```python
from build123d import *

# Parameters (mm, degrees)
BOSS_EXTRUDE2_DEPTH     = 12
CUT_EXTRUDE1_DEPTH      = 13
SKETCH3_R               = 1.25
CUT_EXTRUDE2_DEPTH      = 13
SKETCH5_R               = 1.65
CUT_EXTRUDE3_DEPTH      = 6
SKETCH6_W               = 12
SKETCH6_H               = 6
CUT_EXTRUDE4_DEPTH      = 13
SKETCH8_W               = 64
SKETCH8_H               = 8
BOSS_EXTRUDE3_DEPTH     = 5
SKETCH9_R               = 1.65
CUT_EXTRUDE5_DEPTH      = 5
SKETCH10_R              = 2
CUT_EXTRUDE6_DEPTH      = 2.5
CUT_EXTRUDE7_DEPTH      = 71.896039473
CUT_EXTRUDE7_DEPTH_BACK = 10


with BuildPart() as part:
    # Sketch1 → Boss-Extrude2 (new body)
    with BuildSketch(Plane.XY):
        with BuildLine():
            Line((0, 0), (64, 0))
            Line((64, 0), (71.941945847, 6.076635266))
            Line((71.941945847, 6.076635266), (89.619615377, 23.754304796))
            ThreePointArc((89.619615377, 23.754304796), (95.283552654, 63.552389681), (55.861435714, 71.4177849))
            Line((55.861435714, 71.4177849), (-7.778174593, 7.778174593))
            Line((-7.778174593, 7.778174593), (0, 0))
        make_face()
    extrude(amount=BOSS_EXTRUDE2_DEPTH)

    # Sketch2 → Cut-Extrude1 (cut, through all)
    with BuildSketch(Plane.XY.offset(12)):
        Polygon((56.718479601, 14.889386235), (39.391727984, 32.210866495), (71.348091567, 64.176955192), (88.674843183, 46.855474932), align=None)
    extrude(amount=-CUT_EXTRUDE1_DEPTH, mode=Mode.SUBTRACT)

    # Sketch3 → Cut-Extrude2 (cut, through all)
    with BuildSketch(Plane.XY.offset(12)):
        with Locations((85.317188693, 39.60711951)):
            Circle(SKETCH3_R)
        with Locations((73.296373413, 27.58630423)):
            Circle(SKETCH3_R)
        with Locations((61.275558133, 15.565488949)):
            Circle(SKETCH3_R)
        with Locations((64.100758142, 60.817095339)):
            Circle(SKETCH3_R)
        with Locations((52.083601094, 48.792622939)):
            Circle(SKETCH3_R)
        with Locations((40.066444047, 36.76815054)):
            Circle(SKETCH3_R)
    extrude(amount=-CUT_EXTRUDE2_DEPTH, mode=Mode.SUBTRACT)

    # Sketch5 → Cut-Extrude3 (cut)
    with BuildSketch(Plane.XZ):
        with Locations((11.5, 6)):
            Circle(SKETCH5_R)
        with Locations((52.5, 6)):
            Circle(SKETCH5_R)
    extrude(amount=-CUT_EXTRUDE3_DEPTH, mode=Mode.SUBTRACT)

    # Sketch6 → Cut-Extrude4 (cut, through all)
    with BuildSketch(Plane.XY.offset(12)):
        with Locations((12, 9)):
            Rectangle(SKETCH6_W, SKETCH6_H)
        with Locations((52, 9)):
            Rectangle(SKETCH6_W, SKETCH6_H)
    extrude(amount=-CUT_EXTRUDE4_DEPTH, mode=Mode.SUBTRACT)

    # Sketch8 → Boss-Extrude3 (add)
    with BuildSketch(Plane.XZ):
        with Locations((32, 16)):
            Rectangle(SKETCH8_W, SKETCH8_H)
    extrude(amount=-BOSS_EXTRUDE3_DEPTH)

    # Sketch9 → Cut-Extrude5 (cut)
    with BuildSketch(Plane.XZ):
        with Locations((11.5, 16)):
            Circle(SKETCH9_R)
        with Locations((52.5, 16)):
            Circle(SKETCH9_R)
    extrude(amount=-CUT_EXTRUDE5_DEPTH, mode=Mode.SUBTRACT)

    # Sketch10 → Cut-Extrude6 (cut)
    with BuildSketch(Plane.XY.offset(12)):
        with Locations((85.317188693, 39.60711951)):
            Circle(SKETCH10_R)
        with Locations((73.296373413, 27.58630423)):
            Circle(SKETCH10_R)
        with Locations((61.275558133, 15.565488949)):
            Circle(SKETCH10_R)
        with Locations((40.060741262, 36.78030582)):
            Circle(SKETCH10_R)
        with Locations((52.081556543, 48.8011211)):
            Circle(SKETCH10_R)
        with Locations((64.102371823, 60.82193638)):
            Circle(SKETCH10_R)
    extrude(amount=-CUT_EXTRUDE6_DEPTH, mode=Mode.SUBTRACT)

    # Sketch11 → Cut-Extrude7 (cut, two sides)
    with BuildSketch(Plane(origin=(0, 5, 0), x_dir=(1, 0, 0), z_dir=(0, 1, 0))) as cut_extrude7_sk:
        with BuildLine():
            ThreePointArc((45, -20), (32, -14.615223689), (19, -20))
            Line((19, -20), (45, -20))
        make_face()
    extrude(amount=CUT_EXTRUDE7_DEPTH, mode=Mode.SUBTRACT)
    extrude(cut_extrude7_sk.sketch, amount=-CUT_EXTRUDE7_DEPTH_BACK, mode=Mode.SUBTRACT)


solid = part.part
```
Build history of the part. All positions in model axes, mm. A direction names the side the tool comes from. Give positions to 0.01 mm unless a question says otherwise; leave off trailing zeros. Loops run counter-clockwise (first coordinate to the right, second up) from the corner with the lowest first, then second, coordinate; pieces in that order, holes last.
1) Band-saw the part on B-B on x = 15. List the corners of the cut face in (y, z).
Values follow:
outline: (0, 0) - (6, 0) - (6, 12) - (5, 12) - (5, 20) - (0, 20) - close; (12, 0) - (30.56, 0) - (30.56, 12) - (12, 12) - close
2) Band-saw the part on C-C on z = 6. State how many separate pieces and enclosed holes the cut face has, then the cut area to 3 significant figures.
Values follow:
separate pieces: 1
enclosed holes: 7
area: 3,740 mm2
3) Band-saw the part on D-D on x = 35. List the corners of the cut face in (y, z).
Values follow:
outline: (0, 0) - (50.56, 0) - (50.56, 12) - (5, 12) - (5, 14.86) - (0, 14.86) - close
4) Two-plate mould, pull along Z, no slides. Class faces 1 (the face through (13.024, 2.958, 5.368)), 2 (the face through (60.284, 14.805, 4.816)), 3 (the face through (84, 39, 9.5)): released by +Z, released by -Z, zero draft, split by the parting line, or undercut.
Values follow:
face 1: undercut
face 2: zero draft
face 3: released by +Z
5) 3-axis set-ups, long thin cutter, end or side, ignore diameter. For faces 4 (the face through (50.85, 2.46, 16.07)), 5 (the face through (41, 38, 9.5)), 6 (the face through (18, 9, 6)), 7 (the face through (64, 2, 16)): which of +Z, -Z, +X, -X, +Y, -Y reach the whole face in a straight line?
Values follow:
face 4: +Y, -Y
face 5: +Z
face 6: +Z, -Z
face 7: +Z, +X, +Y, -Y
6) Band-saw the part on A-A on z = 16. List the corners of the cut face in (x, y).
Values follow:
outline: (0, 0) - (9.85, 0) - (9.85, 5) - (0, 5) - close; (13.15, 0) - (25, 0) - (25, 5) - (13.15, 5) - close; (39, 0) - (50.85, 0) - (50.85, 5) - (39, 5) - close; (54.15, 0) - (64, 0) - (64, 5) - (54.15, 5) - close
7) Drop flat-ended pins along their axis: P1, Ø1.5, axis at x = 85.32, y = 39.61, coming from the -Z side; P2, Ø4.5, axis at x = 73.5, y = 28, coming from the +Z side; P3, Ø3, axis at x = 64.1, y = 60.82, coming from the +Z side; P4, Ø3, axis at y = 8, z = 7, coming from the +X side. Give the stop position or say it passes through.
Values follow:
P1: passes through
P2: stops at z = 12
P3: stops at z = 9.5
P4: stops at x = 75.37
8) Probe line 1 along Z through (x, y) = (11.5, 3.75); line 2 along X through (y, z) = (16, 3.75); line 3 along Y through (x, z) = (53, 9.25). List the from-to ranges inside material, lowest first.
Values follow:
line 1: z = 0 to 4.35, 7.65 to 14.35, 17.65 to 20
line 2: x = 0.44 to 55.61, 57.83 to 60.1, 62.45 to 81.87
line 3: y = 0 to 6, 12 to 18.61, 45.82 to 47.94, 49.64 to 68.56
